Input: part model. Units: mm. Frame: model coordinates. A direction names the side the tool comes from. Round coordinates to 2 decimals unless told otherwise and drop trailing zeros. Order: outer loops, then holes, each group sorted by start corner. A loop starts at its lowest first (then second) coordinate and runs counter-clockwise, first axis right, second up. Notation, with made-up numbers: (51.25, 17) - (76.25, 17) arc R21 ccw to (76.25, 50) - close; hole circle Ø5 at (-29, 49). An arc over 180 degrees is marked (long way). One line per item, written item: value. Start each with the question number.
Autodesk Inventor part; units mm, degrees
ref_plane "Work Plane1" through (35.2128, 29.2169, 0) normal (0.5, 0.8660254, 0) x (-0.8660254, 0.5, 0)
ref_plane "Work Plane2" through (37.7128, 24.8868, 0) normal (1, 0, 0) x (0, 1, 0)
ref_plane "YZ Plane" through (0, 0, 0) normal (1, 0, 0) x (0, 1, 0)
sketch "Sketch1" plane through (0, 0, 0) normal (0, 0, 1) x (1, 0, 0)
  line L0 (37.7128, 0) -> (0, 0)
  line L1 (0, 0) -> (34.8308, 60.3287)
  line L2 (27.7128, 0) -> (27.7128, 19.1132)
  line L3 (25.2128, 23.4434) -> (16.4545, 28.5)
  line L4 (37.7128, 0) -> (37.7128, 24.8868)
  line L5 (35.2128, 29.2169) -> (21.4545, 37.1603)
  arc A0 (27.7128, 19.1132) -> (25.2128, 23.4434) centre (22.7128, 19.1132) ccw
  arc A1 (37.7128, 24.8868) -> (35.2128, 29.2169) centre (32.7128, 24.8868) ccw
  line L6 (21.4545, 37.1603) -> (16.4545, 28.5)
  line L7 (21.4545, 37.1603) -> (35.2128, 29.2169)
  line L8 (16.4545, 28.5) -> (25.2128, 23.4434)
  line L9 (27.7128, 0) -> (37.7128, 0)
  line L10 (37.7128, 0) -> (37.7128, 24.8868)
  line L11 (27.7128, 0) -> (37.7128, 0)
  line L12 (37.7128, 0) -> (37.7128, 24.8868)
  line L13 (35.2128, 29.2169) -> (21.4545, 37.1603)
  line L14 (21.4545, 37.1603) -> (16.4545, 28.5)
  line L15 (16.4545, 28.5) -> (25.2128, 23.4434)
  line L16 (27.7128, 19.1132) -> (27.7128, 0)
  point P0 (25, 43.3013)
  point P1 (27.7128, 22)
  dimension "d37" = 60
  dimension "d38" = 10
  dimension "d39" = 10
  dimension "d40" = 0
  dimension "d41" = 0
  dimension "d42" = 22
  dimension "d43" = 13
  dimension "d44" = 120
  dimension "d45" = 5
extrude "Extrusion1" add sketch "Sketch1" along normal blind 12 contours L0 L2 A0 L3 L1 L5 A1 L4
ref_plane "Work Plane1" through (35.2128, 29.2169, 0) normal (0.5, 0.8660254, 0) x (-0.8660254, 0.5, 0)
sketch "Sketch2" plane through (35.2128, 29.2169, 0) normal (0.5, 0.8660254, 0) x (-0.8660254, 0.5, 0)
  circle A0 centre (15.8868, 6) radius 6
  line L0 (15.8868, 0) -> (15.8868, 12)
  line L1 (0, 12) -> (15.8868, 12)
  dimension "d5" = 12
  dimension "d47" = 0
  dimension "d48" = 6
extrude "Extrusion2" add sketch "Sketch2" against normal blind 10
ref_plane "Work Plane2" through (37.7128, 24.8868, 0) normal (1, 0, 0) x (0, 1, 0)
sketch "Sketch3" plane through (37.7128, 24.8868, 0) normal (1, 0, 0) x (0, 1, 0)
  circle A0 centre (-24.8868, 6) radius 6
  line L0 (-24.8868, 0) -> (-24.8868, 12)
  line L1 (-24.8868, 0) -> (0, 0)
  point P0 (43.3013, 10)
  point P1 (3.6132, 12)
  dimension "d10" = 12
  dimension "d49" = 0
  dimension "d50" = 6
extrude "Extrusion3" add sketch "Sketch3" against normal blind 10
sketch "Sketch4" plane through (30.2128, 20.5566, 0) normal (-0.5, -0.8660254, 0) x (0.8660254, -0.5, 0)
  circle A0 centre (-15.8868, 6) radius 2.5
  circle A1 centre (-15.8868, 6) radius 6
  point P0 (-15.8868, 0)
  point P1 (-15.8868, 12)
  dimension "d15" = 5
extrude "Extrusion4" cut sketch "Sketch4" along normal through all both and the other way through all contours A0
sketch "Sketch5" plane through (27.7128, 24.8868, 0) normal (-1, 0, 0) x (0, 0, 1)
  circle A0 centre (6, -24.8868) radius 2.5
  arc A1 (0, -24.8868) -> (12, -24.8868) centre (6, -24.8868) ccw
  dimension "d18" = 5
extrude "Extrusion5" cut sketch "Sketch5" along normal through all both and the other way through all
sketch "Sketch6" plane through (35.2128, 29.2169, 0) normal (0.5, 0.8660254, 0) x (0.8660254, -0.5, 0)
  circle A0 centre (-15.8868, -6) radius 3.6
  circle A1 centre (-15.8868, -6) radius 2.5
  arc A2 (-15.8868, 0) -> (-15.8868, 0) centre (-15.8868, -6) ccw
  point P0 (0, -10)
  dimension "d21" = 5
  dimension "d22" = 7.2
extrude "Extrusion6" cut sketch "Sketch6" against normal blind 3 contours A0
sketch "Sketch7" plane through (30.2128, 20.5566, 0) normal (-0.5, -0.8660254, 0) x (0.8660254, -0.5, 0)
  circle A0 centre (-15.8868, 6) radius 3.6
  circle A1 centre (-15.8868, 6) radius 2.5
  arc A2 (-13.3868, 6) -> (-13.3868, 6) centre (-15.8868, 6) ccw
  point P0 (-15.8868, 0)
  dimension "d25" = 5
  dimension "d26" = 7.2
extrude "Extrusion7" cut sketch "Sketch7" along normal mid plane 6
sketch "Sketch8" plane through (27.7128, 24.8868, 0) normal (-1, 0, 0) x (0, 0, 1)
  circle A0 centre (6, -24.8868) radius 3.6
  circle A1 centre (6, -24.8868) radius 2.5
  arc A2 (8.5, -24.8868) -> (8.5, -24.8868) centre (6, -24.8868) ccw
  point P0 (0, -24.8868)
  dimension "d29" = 7.2
  dimension "d30" = 5
extrude "Extrusion8" cut sketch "Sketch8" along normal mid plane 6
sketch "Sketch9" plane through (37.7128, 24.8868, 0) normal (1, 0, 0) x (0, 0, -1)
  circle A0 centre (-6, -24.8868) radius 3.6
  circle A1 centre (-6, -24.8868) radius 2.5
  circle A2 centre (-6, -24.8868) radius 2.5
  point P0 (0, -24.8868)
  dimension "d33" = 5
  dimension "d34" = 7.2
extrude "Extrusion9" cut sketch "Sketch9" against normal blind 3
fillet "Fillet1" radius 2 16 edges at (16.2583, 40.1603, 6) (28.3336, 33.1886, 0) (37.0429, 27.3868, 0) (37.7128, 12.4434, 0) (37.7128, -6, 6) (37.7128, 12.4434, 12) (37.0429, 27.3868, 12) (28.3336, 33.1886, 12) (27.0429, 21.6132, 12) (27.7128, 9.5566, 12) (27.7128, -6, 6) (27.7128, 9.5566, 0) (27.0429, 21.6132, 0) (20.8336, 25.9717, 0) (11.2583, 31.5, 6) (20.8336, 25.9717, 12)
equation "\"d38\" = d46"
equation "\"d39\" = d46"
equation "\"d3\" = width"
equation "\"d5\" = width"
equation "\"d48\" = 0.5 * width"
equation "\"d8\" = thickness"
equation "\"d10\" = width"
equation "\"d50\" = 0.5 * width"
equation "\"d13\" = thickness"
equation "\"thickness\" = thickness_1"
equation "\"width\" = width_1"
equation "\"d46\" = 10"
properties part number "Link2"
Item 1: First-contact query: pin 1 Ø4 at (y, z) = (4, 5) entering from -X; pin 2 Ø2 at (y, z) = (0.5, 5) entering from -X; pin 3 Ø6.5 at (y, z) = (0, 6) entering from +X; pin 4 Ø4 at (x, z) = (23.5, 8) entering from +Y. Flat tips, straight axial feed; report the tip coordinate or a pass-through.
Item 2: Pull-direction query (X, two-part tool) for faces 4 (the face through (37.024, 27.418, 5.944)), 5 (the face through (19.297, 30.325, 3.65)), 6 (the face through (30.713, 0.9, 3.5)); classes: released by +X, released by -X, zero draft, split by the parting line, or undercut.
Item 3: Line query: L1, parallel to Y at x = 29.4, z = 6; L2, parallel to Y at x = 33.3, z = 6; L3, parallel to X at y = 14, z = 6.75. Output: solid intervals per line, ascending.
Item 4: Section query B-B on z = 6. Give the number of separate pieces and of enclosed holes in the cut face, and give its area (3 significant figures).
Item 5: Reachability of faces 1 (the face through (34.713, 0.9, 8.5)), 2 (the face through (27.713, 10, 6)), 3 (the face through (28.283, 9.69, 11.399)) from +Z, -Z, +X, -X, +Y, -Y: full face, straight path, thin tool, end or side. Return the list, or none.
Item 6: Section query A-A on y = 15. Return loops of the section in (x, z), and give its area (3 significant figures).
Geometry results:
1. pin 1: stops at x = 27.71
1. pin 2: passes through
1. pin 3: stops at x = 34.71
1. pin 4: stops at y = 36.74
2. face 4: released by +X
2. face 5: undercut
2. face 6: released by -X
3. L1: y = -5.98 to -3.6, 3.6 to 32.57
3. L2: y = -6 to -2.5, 2.5 to 30.32
3. L3: x = 27.71 to 37.71
4. separate pieces: 3
4. enclosed holes: 0
4. area: 398 mm^2
5. face 1: +X
5. face 2: +Z, -Z, -X, -Y
5. face 3: +Z, -X, -Y
6. outline: (27.71, 2) arc R2 ccw to (29.71, 0) - (35.71, 0) arc R2 ccw to (37.71, 2) - (37.71, 10) arc R2 ccw to (35.71, 12) - (29.71, 12) arc R2 ccw to (27.71, 10) - close
6. area: 117 mm^2
